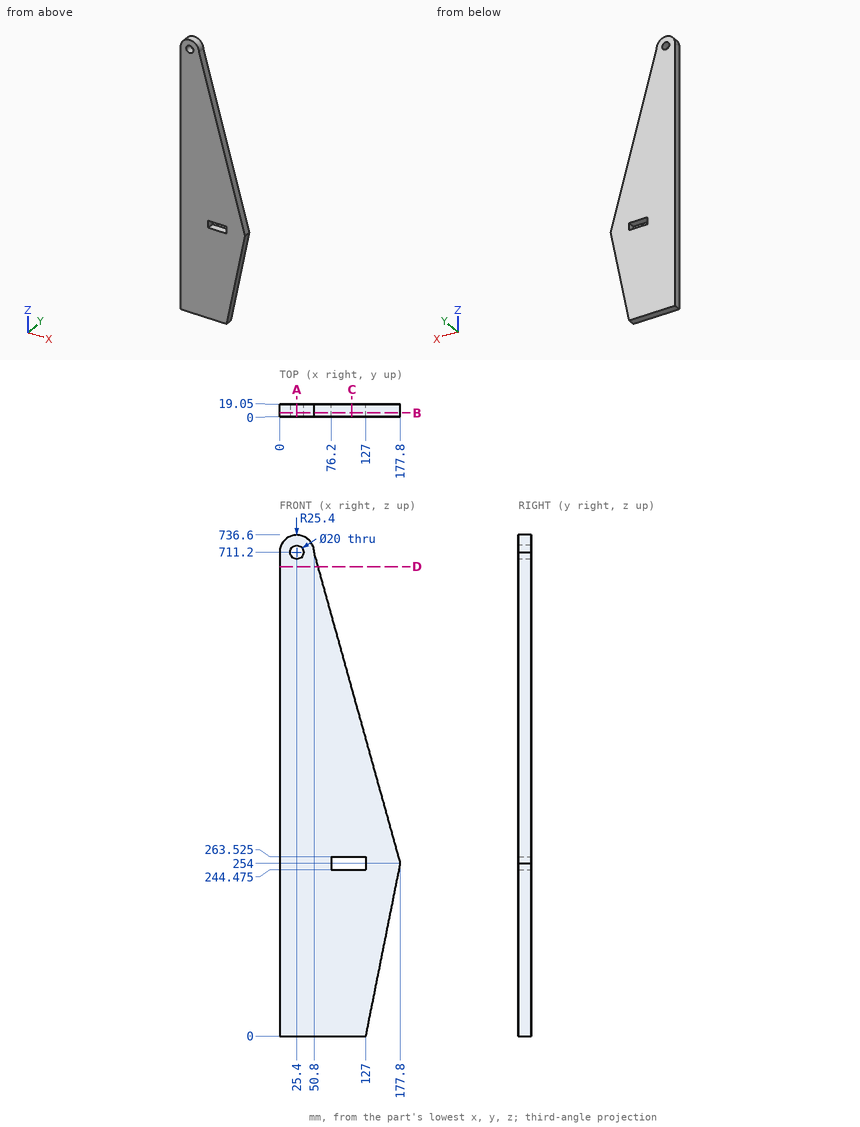
Geometry: see drawing. Coordinates: mm, zero at the bounding-box minimum. Give positions to 0.01 mm unless a question says otherwise; leave off trailing zeros. Order: outer loops, then holes, each group sorted by start corner. A loop starts at its lowest first (then second) coordinate and runs counter-clockwise, first axis right, second up. Notation, with made-up numbers: (82, -36.5) - (110, -36.5) arc R16 cw to (110, -12.5) - close; hole circle Ø1 at (-23.5, -25). An arc over 180 degrees is marked (long way). Write each question's results on one line, items separated by ' | '.
Item 1: Material intervals for line 1 along Z through (x, y) = (25.4, 7.5); line 2 along X through (y, z) = (9.5, 711.2); line 3 along X through (y, z) = (5.75, 532), sorted ascending.
A:
line 1: z = 0 to 701.2, 721.2 to 736.6 | line 2: x = 0 to 15.4, 35.4 to 50.8 | line 3: x = 0 to 100.58
Item 2: Section C-C (x = 106.5). Return loops of the section in (y, z) (3 decimals), and give its area (3 significant figures).
A:
outline: (0, 0) - (19.05, 0) - (19.05, 244.475) - (0, 244.475) - close; (0, 263.525) - (19.05, 263.525) - (19.05, 510.68) - (0, 510.68) - close | area: 9,370 mm^2
Item 3: Section A-A (x = 25.4). Return loops of the section in (y, z).
A:
outline: (0, 0) - (19.05, 0) - (19.05, 701.2) - (0, 701.2) - close; (0, 721.2) - (19.05, 721.2) - (19.05, 736.6) - (0, 736.6) - close
Item 4: Section B-B (y = 6). Return loops of the section in (x, z) (3 decimals).
A:
outline: (0, 0) - (127, 0) - (177.8, 254) - (50.8, 711.2) arc R25.4 ccw to (0, 711.2) - close; hole circle Ø20 at (25.4, 711.2); hole (76.2, 244.475) - (127, 244.475) - (127, 263.525) - (76.2, 263.525) - close
Item 5: Section D-D (z = 690). Return loops of the section in (x, y), and give its area (3 significant figures).
A:
outline: (0, 0) - (56.69, 0) - (56.69, 19.05) - (0, 19.05) - close | area: 1,080 mm^2
